Input: part model. Units: mm. Frame: model coordinates. A direction names the side the tool comes from. Round coordinates to 2 decimals unless told otherwise and drop trailing zeros. Loops run counter-clockwise (first coordinate to the right, second up) from the corner with the lowest first, then second, coordinate; pieces in that order, holes last. Notation, with made-up numbers: M 33,-5 L 70,-5 A22 cw 70,32 Z; hole C 13,-31 d10. An arc over 180 degrees is marked long. Put each result on its own line as item: value. Start each with the question number.
1) Draft query along Y for faces 5 (the face through (25, 122, 5)), 6 (the face through (127.86, 0.9, 4.93)), 7 (the face through (120, 30, 5)). Return one class per face: +Y half, -Y half, draft (parallel to the pull), parting line (faces both ways), or undercut.
2) Section B-B on x = -74. Output: boundary loops of the cut face in (y, z).
3) Section A-A on y = 35.5. Output: boundary loops of the cut face in (x, z).
4) Section C-C on z = 7.75. State how many separate pieces and enclosed holes the cut face has, plus the area to 3 significant figures.
5) Pin query (flat end, axial travel): pin 1 (5 mm diameter, centred on y = 124, z = 7.5, fed in from -X); pin 2 (8 mm diameter, centred on x = 93.5, y = 63, fed in from +Z); pin 3 (1 mm diameter, centred on x = -45.5, z = 8.5, fed in from +Y); pin 4 (4 mm diameter, centred on x = 80.5, z = 8, fed in from -Y). Return the tip coordinate at first contact, or that it passes through.
6) Line query: probe 1 along X at (y, z) = (-82, 7); probe 2 along Y at (x, z) = (-105.5, 1.5); probe 3 along X at (y, z) = (130.5, 3.85). Output: solid intervals per line, ascending.
7) Reachability of faces 1 (the face through (25, -123, 5)), 2 (the face through (105, 50, 5)), 3 (the face through (-3, 117, 6)), 4 (the face through (-25, -122, 5)) from +Z, -Z, +X, -X, +Y, -Y: full face, straight path, thin tool, end or side. Return the list, or none.
from build123d import *

# Parameters (mm, degrees)
SKETCH_R     = 60
SKETCH_R_2   = 3
SKETCH_R_3   = 8
SKETCH_R_4   = 1.75
SKETCH_R_5   = 5.75
SKETCH_R_6   = 1.5
PAD_DEPTH    = 10
SKETCH001_R  = 11.75
POCKET_DEPTH = 4
FILLET_R     = 5


with BuildPart() as part:
    # Sketch → Pad (new body)
    with BuildSketch(Plane.XY):
        Polygon((-105, 70), (-105, 30), (-135, 30), (-135, -30), (-105, -30), (-105, -70), (-140, -70), (-140, -105), (-105, -105), (-25, -105), (-25, -140), (25, -140), (25, -105), (105, -105), (140, -105), (140, -70), (105, -70), (105, -30), (135, -30), (135, 30), (105, 30), (105, 70), (140, 70), (140, 105), (105, 105), (25, 105), (25, 140), (-25, 140), (-25, 105), (-105, 105), (-140, 105), (-140, 70), align=None)
        Circle(SKETCH_R, mode=Mode.SUBTRACT)
        with Locations((93.5, 95)):
            Circle(SKETCH_R_2, mode=Mode.SUBTRACT)
        with Locations((93.5, 63)):
            Circle(SKETCH_R_2, mode=Mode.SUBTRACT)
        with Locations((93.5, -63)):
            Circle(SKETCH_R_2, mode=Mode.SUBTRACT)
        with Locations((93.5, -95)):
            Circle(SKETCH_R_2, mode=Mode.SUBTRACT)
        with Locations((-93.5, -63)):
            Circle(SKETCH_R_2, mode=Mode.SUBTRACT)
        with Locations((-93.5, -95)):
            Circle(SKETCH_R_2, mode=Mode.SUBTRACT)
        with Locations((-93.5, 95)):
            Circle(SKETCH_R_2, mode=Mode.SUBTRACT)
        with Locations((-93.5, 63)):
            Circle(SKETCH_R_2, mode=Mode.SUBTRACT)
        with Locations((122.5, 87.5)):
            Circle(SKETCH_R_3, mode=Mode.SUBTRACT)
        with Locations((122.5, -87.5)):
            Circle(SKETCH_R_3, mode=Mode.SUBTRACT)
        with Locations((-122.5, -87.5)):
            Circle(SKETCH_R_3, mode=Mode.SUBTRACT)
        with Locations((-122.5, 87.5)):
            Circle(SKETCH_R_3, mode=Mode.SUBTRACT)
        with Locations((125, 20)):
            Circle(SKETCH_R_2, mode=Mode.SUBTRACT)
        with Locations((125, 0)):
            Circle(SKETCH_R_2, mode=Mode.SUBTRACT)
        with Locations((125, -20)):
            Circle(SKETCH_R_2, mode=Mode.SUBTRACT)
        with Locations((-125, 20)):
            Circle(SKETCH_R_2, mode=Mode.SUBTRACT)
        with Locations((-125, 0)):
            Circle(SKETCH_R_2, mode=Mode.SUBTRACT)
        with Locations((-125, -20)):
            Circle(SKETCH_R_2, mode=Mode.SUBTRACT)
        with Locations((110.124738, -75.124738)):
            Circle(SKETCH_R_4, mode=Mode.SUBTRACT)
        with Locations((134.873476, -99.873476)):
            Circle(SKETCH_R_4, mode=Mode.SUBTRACT)
        with Locations((110.124738, 75.124738)):
            Circle(SKETCH_R_4, mode=Mode.SUBTRACT)
        with Locations((134.873476, 99.873476)):
            Circle(SKETCH_R_4, mode=Mode.SUBTRACT)
        with Locations((-110.124738, 75.124738)):
            Circle(SKETCH_R_4, mode=Mode.SUBTRACT)
        with Locations((-134.873476, 99.873476)):
            Circle(SKETCH_R_4, mode=Mode.SUBTRACT)
        with Locations((-110.124738, -75.124738)):
            Circle(SKETCH_R_4, mode=Mode.SUBTRACT)
        with Locations((-134.873476, -99.873476)):
            Circle(SKETCH_R_4, mode=Mode.SUBTRACT)
        with Locations((0, 122.5)):
            Circle(SKETCH_R_5, mode=Mode.SUBTRACT)
        with Locations((0, -122.5)):
            Circle(SKETCH_R_5, mode=Mode.SUBTRACT)
        with Locations((8, -122.5)):
            Circle(SKETCH_R_6, mode=Mode.SUBTRACT)
        with Locations((0, -114.5)):
            Circle(SKETCH_R_6, mode=Mode.SUBTRACT)
        with Locations((-8, -122.5)):
            Circle(SKETCH_R_6, mode=Mode.SUBTRACT)
        with Locations((0, -130.5)):
            Circle(SKETCH_R_6, mode=Mode.SUBTRACT)
        with Locations((0, 130.5)):
            Circle(SKETCH_R_6, mode=Mode.SUBTRACT)
        with Locations((8, 122.5)):
            Circle(SKETCH_R_6, mode=Mode.SUBTRACT)
        with Locations((0, 114.5)):
            Circle(SKETCH_R_6, mode=Mode.SUBTRACT)
        with Locations((-8, 122.5)):
            Circle(SKETCH_R_6, mode=Mode.SUBTRACT)
    extrude(amount=PAD_DEPTH)

    # Sketch001 (on Face63 of Pad) → Pocket (cut)
    with BuildSketch(Plane.XY.offset(10)):
        with Locations((0, 122.5)):
            Circle(SKETCH001_R)
        with Locations((0, -122.5)):
            Circle(SKETCH001_R)
    extrude(amount=-POCKET_DEPTH, mode=Mode.SUBTRACT)

    # Fillet
    fillet_edges = [part.edges().sort_by_distance(p)[0] for p in [
        (25, -105, 5),
        (25, -140, 5),
        (-25, -140, 5),
        (-25, -105, 5),
        (-140, -105, 5),
        (-140, -70, 5),
        (-140, 70, 5),
        (-140, 105, 5),
        (-25, 105, 5),
        (-25, 140, 5),
        (25, 140, 5),
        (25, 105, 5),
        (140, 105, 5),
        (140, 70, 5),
        (140, -70, 5),
        (140, -105, 5),
    ]]
    fillet(fillet_edges, radius=FILLET_R)


solid = part.part
Geometry results:
1. face 5: draft
1. face 6: undercut
1. face 7: undercut
2. outline: M -105,0 L 105,0 L 105,10 L -105,10 Z
3. outline: M -105,0 L -48.37,0 L -48.37,10 L -105,10 Z; M 48.37,0 L 105,0 L 105,10 L 48.37,10 Z
4. separate pieces: 1
4. enclosed holes: 29
4. area: 42,600 mm²
5. pin 1: stops at x = -25
5. pin 2: stops at z = 10
5. pin 3: stops at y = 105
5. pin 4: stops at y = -105
6. probe 1: x = -140 to -128.31, -116.69 to 116.69, 128.31 to 140
6. probe 2: y = -105 to -70, -30 to 30, 70 to 105
6. probe 3: x = -25 to -1.5, 1.5 to 25
7. face 1: +Z, -Z, +X, -Y
7. face 2: +Z, -Z, +X
7. face 3: +Z
7. face 4: +Z, -Z, -X, -Y
